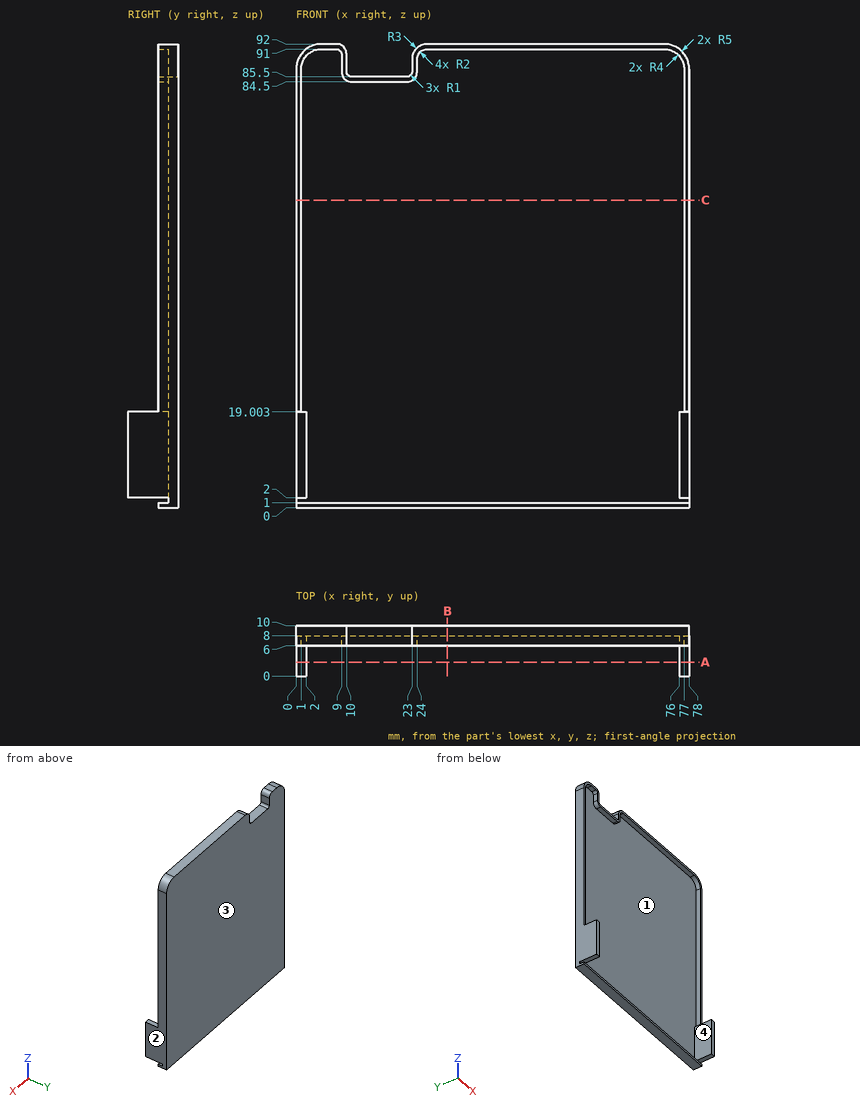
Design review of the part shown in the three views and the two pictorial views. Dimensions are in mm from the part's minimum x, y and z. Round coordinates to 2 decimals unless told otherwise and drop trailing zeros. Order: outer loops, then holes, each group sorted by start corner. A loop starts at its lowest first (then second) coordinate and runs counter-clockwise, first axis right, second up. Notation, with made-up numbers: (-27.75, 46) - (-16.75, 46) arc R19 cw to (-16.75, 82) - close; hole circle Ø10 at (59.5, 11). An arc over 180 degrees is marked (long way). One line per question, with ' | ' between items.
Item 1: Take a section at A-A, the plane y = 2.75. Write out the cut boundary in (x, z), then the cut area to 3 significant figures.
Checks:
outline: (0, 2) - (2, 2) - (2, 19) - (0, 19) - close; (76, 2) - (78, 2) - (78, 19) - (76, 19) - close | area: 68.0 mm²
Item 2: Draft analysis for pull direction X (two halves, no side actions). For the marked faces 1, 2, 3 and 4, state which applies: +X half, -X half, draft (parallel to the pull), parting line (faces both ways), or undercut.
Checks:
face 1: undercut | face 2: +X half | face 3: draft | face 4: undercut
Item 3: For P1, Ø2.5, axis at y = 2, z = 11, coming from the -X side; P2, Ø0.6, axis at x = 1, y = 5, coming from the +Z side; P3, Ø3, axis at x = 15, z = 79, coming from the -Y side; P4, Ø3, axis at x = 15.5, y = 8.5, coming from the +Z side, all flat-tipped, find the tip position at first contact; note any pin that passes through.
Checks:
P1: x = 0 | P2: z = 19 | P3: y = 8 | P4: z = 85.5
Item 4: Take a section at C-C, the plane z = 61. Write out the cut boundary in (x, y).
Checks:
outline: (0, 6) - (1, 6) - (1, 8) - (77, 8) - (77, 6) - (78, 6) - (78, 10) - (0, 10) - close
Item 5: Wall thickness on line 1 (Z direction, x = 70, y = 7); line 2 (X direction, y = 6.5, z = 30.5); line 3 (Y direction, x = 26.5, z = 85.5): over which ranges is each line inside the solid? List them lowest first. Write a range as [from, to].
Checks:
line 1: [0, 1], [91, 92] | line 2: [0, 1], [77, 78] | line 3: [8, 10]
Item 6: Take a section at B-B, the plane x = 30. Write out the cut boundary in (y, z), then the cut area to 3 significant figures.
Checks:
outline: (6, 0) - (10, 0) - (10, 92) - (6, 92) - (6, 91) - (8, 91) - (8, 1) - (6, 1) - close | area: 188 mm²
